Check sheet for the drawn part. Datum: minimum x, y, z corner. Units: mm. A direction names the side the tool comes from. Give positions to 0.01 mm unless a question says otherwise; leave off trailing zeros. Loops run counter-clockwise (first coordinate to the right, second up) from the corner with the lowest first, then second, coordinate; pieces in that order, holes last. Notation, with made-up numbers: (-20.75, -5.5) - (23.25, -5.5) arc R8 ccw to (23.25, 9.5) - close; hole circle Ø8 at (52, -18). An arc over 180 degrees is marked (long way). Use one line per item in the form item = value.
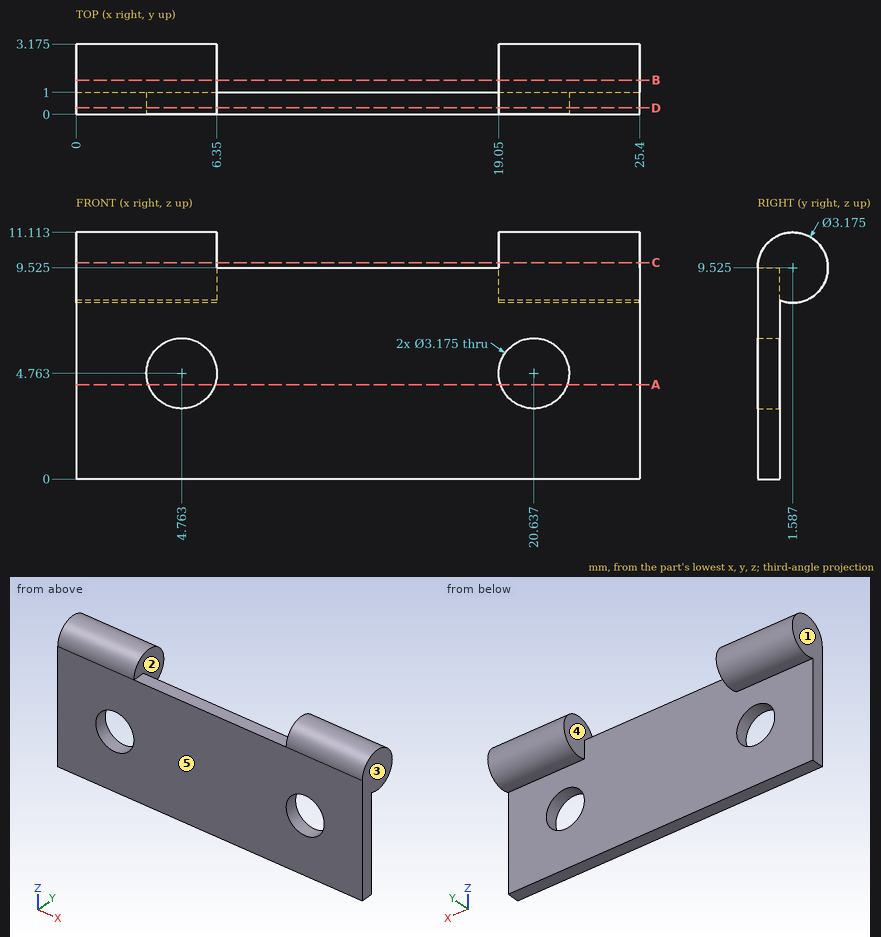
Item 1: Section check B-B on y = 1.55. Record the boundary of the cut face in (x, z).
Answer block:
outline = (0, 7.94) - (6.35, 7.94) - (6.35, 11.11) - (0, 11.11) - close; (19.05, 7.94) - (25.4, 7.94) - (25.4, 11.11) - (19.05, 11.11) - close
Item 2: Access from +Z, -Z, +X, -X, +Y, -Y to the whole of each face (thin tool, end or side, straight path). Record for the marked faces 4 and 5.
Answer block:
face_4 = +Z, +Y
face_5 = +Z, -Z, +X, -X, -Y
Item 3: Section check A-A on z = 4.25. Record the boundary of the cut face in (x, y) (1 decimal).
Answer block:
outline = (0, 0) - (3.3, 0) - (3.3, 1) - (0, 1) - close; (6.3, 0) - (19.1, 0) - (19.1, 1) - (6.3, 1) - close; (22.1, 0) - (25.4, 0) - (25.4, 1) - (22.1, 1) - close
Item 4: Thickness scan on L1, parallel to X at y = 1.8, z = 9.75; L2, parallel to X at y = 0.2, z = 4.25 (1 decimal); L3, parallel to Y at x = 17.5, z = 8.5. Record the ranges inside material, lowest first.
Answer block:
L1 = 0 to 6.35, 19.05 to 25.4
L2 = 0 to 3.3, 6.3 to 19.1, 22.1 to 25.4
L3 = 0 to 1
Item 5: Mould release check, pull along X, two halves, no side actions. Record for the marked faces 1, 2 and 3: released by +X, released by -X, zero draft, split by the parting line, or undercut.
Answer block:
face_1 = released by -X
face_2 = undercut
face_3 = released by +X
Item 6: Gauge pin test, flat ends, axial feed: P1, Ø3, axis at x = 13.5, z = 2.5, coming from the +Y side; P2, Ø2.5, axis at x = 4.76, z = 4.76, coming from the +Y side; P3, Ø0.8, axis at x = 14, y = 0.5, coming from the +Z side (1 decimal). Record the tip position at first contact, or that the pin passes through.
Answer block:
P1 = 1
P2 = through
P3 = 9.5
Item 7: Section check D-D on y = 0.3. Give the number of separate pieces and of enclosed holes in the cut face, then the cut area to 3 significant figures.
Answer block:
separate_pieces = 1
enclosed_holes = 2
area = 238 mm2
Item 8: Section check C-C on z = 9.75. Record the boundary of the cut face in (x, y).
Answer block:
outline = (0, 0.02) - (6.35, 0.02) - (6.35, 3.16) - (0, 3.16) - close; (19.05, 0.02) - (25.4, 0.02) - (25.4, 3.16) - (19.05, 3.16) - close
